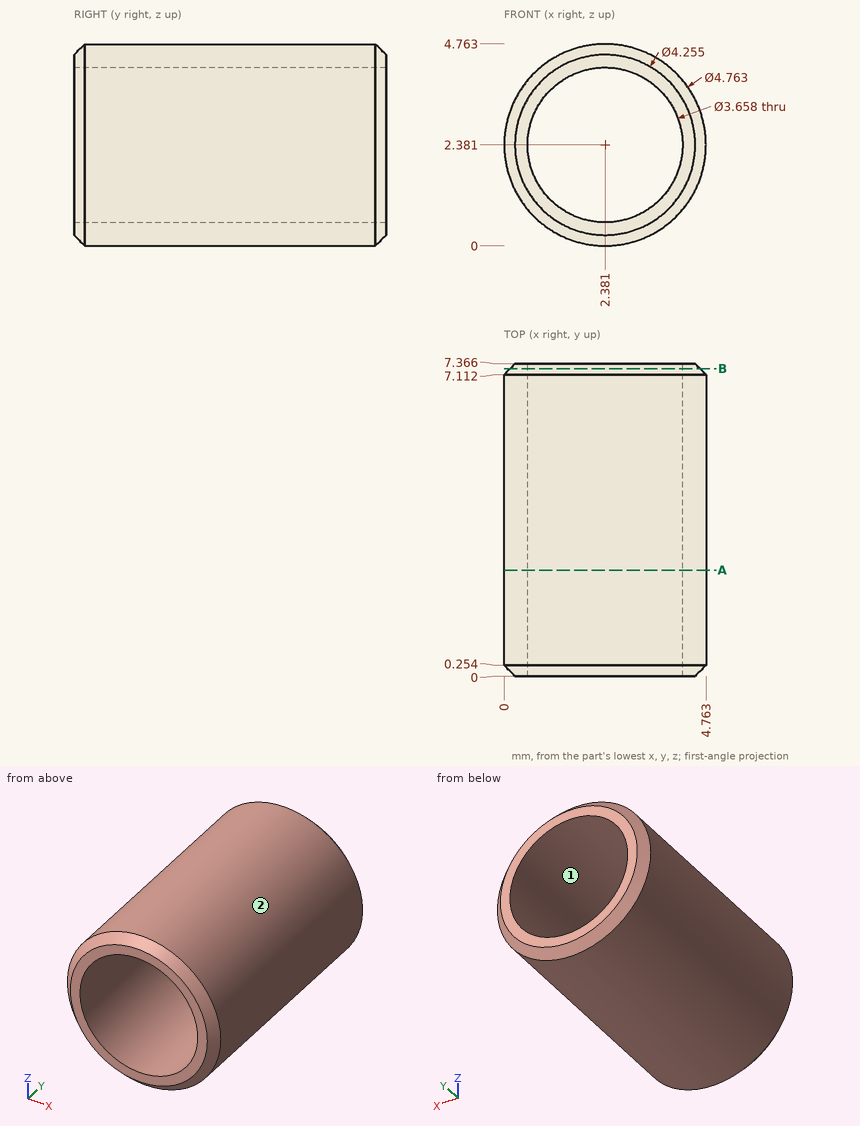
The figure shows three views and two pictorial views of one solid part (mm, origin at its lowest corner). Answer the questions. Round coordinates to 2 decimals unless told otherwise and drop trailing zeros. Write each loop counter-clockwise with the first axis right and the second up, starting at its lowest first coordinate (ties: lowest second). Pieces come first, ordered by that corner, then holes. Notation, with made-up numbers: M 34.5,70 L 47.5,70 A23 ccw 47.5,106 Z; hole C 29,14.25 d6. An arc over 180 degrees is marked long. Use a Markdown table: item, result.
1) Consider line 1 (Z direction, x = 2.3, y = 2.25) (1 decimal); line 2 (Z direction, x = 1.7, y = 4.5) (1 decimal); line 3 (X direction, y = 5.25, z = 3.3) (1 decimal). Determine where each line is inside the solid, lowest interval first. Write a range as [from, to].
Taken from the geometry:
| item | result |
|---|---|
| line 1 | z = [0, 0.6], [4.2, 4.8] |
| line 2 | z = [0.1, 0.7], [4.1, 4.7] |
| line 3 | x = [0.2, 0.8], [4, 4.6] |
2) The part is cut by section B-B on y = 7.25. Give the vertices of the cut face in (x, z) (1 decimal).
Taken from the geometry:
| item | result |
|---|---|
| outline | C 2.4,2.4 d4.5; hole C 2.4,2.4 d3.7 |
3) Flat-ended cylindrical pins translate along their axes: pin 1 (1.5 mm diameter, centred on x = 1.5, y = 2, fed in from +Z); pin 2 (1 mm diameter, centred on x = 1, y = 1, fed in from +Z). Find the tip coordinate at first contact, or state that the pin passes through.
Taken from the geometry:
| item | result |
|---|---|
| pin 1 | stops at z = 4.76 |
| pin 2 | stops at z = 4.59 |
4) Determine the mould class of the marked faces 1 and 2 for opening direction Z: pulls with the +Z half, pulls with the -Z half, needs draft (parallel to the pull), parting line crosses it, or undercut.
Taken from the geometry:
| item | result |
|---|---|
| face 1 | undercut |
| face 2 | parting line crosses it |
5) The part is cut by section A-A on y = 2.5. Give the vertices of the cut face in (x, z).
Taken from the geometry:
| item | result |
|---|---|
| outline | C 2.38,2.38 d4.76; hole C 2.38,2.38 d3.66 |
